Design review of the part built by this model. Coordinates are the model's own, in mm. A direction names the side the tool comes from. Round coordinates to 2 decimals unless told otherwise and drop trailing zeros. Loops run counter-clockwise (first coordinate to the right, second up) from the corner with the lowest first, then second, coordinate; pieces in that order, holes last. Notation, with made-up numbers: (-16.75, 65) - (5.25, 65) arc R32 cw to (5.25, 103) - close; hole circle Ø5 at (-1, 3). An arc over 180 degrees is marked (long way). Answer as CSV lines item,"result". Start each with the question number.
(1) Consider section A-A (z = -13.5). Give the boundary of the cut face in (x, y).
(2) For P1, Ø1.5, axis at x = 1.5, z = 3, coming from the +Y side; P2, Ø3, axis at y = 8.5, z = -5.5, coming from the -X side; P3, Ø1, axis at x = 2, y = -10.5, coming from the +Z side, all flat-tipped, find the tip position at first contact; note any pin that passes through.
(3) For faces 1 (the cylindrical face through (1.726, 1.21, -14.815)), 2 (the cylindrical face through (1.726, -14.464, 3.427)), 3 (the cylindrical face through (2, -14, 6)), 4 (the cylindrical face through (2, 6, 14)), list the 3-axis set-ups (+Z, -Z, +X, -X, +Y, -Y) from which the entire face can be reached by the end or side of a thin tool; tool diameter is ignored.
(4) Consider section C-C (z = 6). Give the boundary of the cut face in (x, y), and give its area (3 significant figures).
(5) Wall thickness on L1, parallel to Y at x = 1.8, z = 14; L2, parallel to Z at x = 3.1, y = -11: over which ranges is each line inside the solid? List them lowest first.
(6) Mouldability with a two-part tool opening along Y and no side actions: class faces 5 (the cylindrical face through (2, -14, -6)), 6 (the cylindrical face through (1.73, 7.74, -12.75)) as released by +Y, released by -Y, zero draft, split by the parting line, or undercut.
(7) Consider section B-B (y = -14). Give the boundary of the cut face in (x, z), and give its area (3 significant figures).
(8) Consider section D-D (y = -9.5). Give the boundary of the cut face in (x, z).
from build123d import *

# Parameters (mm, degrees)
BASPROSKE_W        = 3.5
BASPROSKE_H        = 16.5
TOOTHCUT_DEPTH     = 24.595550428
TEETHCUTS_COUNT    = 20
TEETHCUTS_ANGLE    = 342
BORSKE_R           = 0.5
BORE_DEPTH         = 50.0000508
CUT_EXTRUDE1_DEPTH = 10


with BuildPart() as part:
    # BasProSke → Base-Revolve (revolve)
    with BuildSketch(Plane(origin=(0, 0, 0), x_dir=(1, 0, 0), z_dir=(0, 1, 0)), mode=Mode.PRIVATE) as base_revolve_sk:
        with Locations((1.75, 8.25)):
            Rectangle(BASPROSKE_W, BASPROSKE_H)
    revolve(base_revolve_sk.sketch.rotate(Axis((-10, 0, 0), (1, 0, 0)), 180), axis=Axis((-10, 0, 0), (1, 0, 0)))

    # TooCutSke → ToothCut (cut, through all)
    with BuildSketch(Plane(origin=(0, 0, 0), x_dir=(0, 0, -1), z_dir=(1, 0, 0))):
        with BuildLine():
            ThreePointArc((0.74381438, 13.102904875), (0, 13.124), (-0.74381438, 13.102904875))
            ThreePointArc((-0.74381438, 13.102904875), (-1.226473103, 14.852072512), (-2.209965745, 16.376962373))
            ThreePointArc((-2.209965745, 16.376962373), (0, 16.5254), (2.209965745, 16.376962373))
            ThreePointArc((2.209965745, 16.376962373), (1.226473103, 14.852072512), (0.74381438, 13.102904875))
        make_face()
    toothcut = extrude(amount=TOOTHCUT_DEPTH, mode=Mode.SUBTRACT)

    # TeethCuts: ToothCut ×20 about axis
    teethcuts_axis = Axis((-10, 0, 0), (1, 0, 0))
    for i in range(1, TEETHCUTS_COUNT):
        add(toothcut.rotate(teethcuts_axis, i * TEETHCUTS_ANGLE / (TEETHCUTS_COUNT - 1)), mode=Mode.SUBTRACT)

    # BorSke → Bore (cut, symmetric)
    with BuildSketch(Plane(origin=(0, 0, 0), x_dir=(0, 0, -1), z_dir=(1, 0, 0))):
        with Locations(Location((0, 0, 0), (0, 0, 180))):
            Circle(BORSKE_R)
    extrude(amount=BORE_DEPTH, both=True, mode=Mode.SUBTRACT)

    # Sketch1 → Cut-Extrude1 (cut)
    with BuildSketch(Plane.ZY):
        Polygon((-1.083959973, 0.232340082), (-1.46991278, -0.097897743), (-1.664721638, 0.37121429), (-2.099317612, 0.190738968), (-1.908578644, 0), (-2.267755891, -0.359177248), (-1.815166156, -0.589783236), (-2.045772144, -1.042372971), (-1.544072558, -1.12183438), (-1.623533966, -1.623533966), (-1.12183438, -1.544072558), (-1.042372971, -2.045772144), (-0.589783236, -1.815166156), (-0.359177248, -2.267755891), (0, -1.908578644), (0.359177248, -2.267755891), (0.589783236, -1.815166156), (1.042372971, -2.045772144), (1.12183438, -1.544072558), (1.623533966, -1.623533966), (1.544072558, -1.12183438), (2.045772144, -1.042372971), (1.815166156, -0.589783236), (2.267755891, -0.359177248), (1.908578644, 0), (2.267755891, 0.359177248), (1.815166156, 0.589783236), (2.045772144, 1.042372971), (1.544072558, 1.12183438), (1.623533966, 1.623533966), (1.182876639, 1.553740702), (0.828023136, 1.406380155), (1.022831994, 0.937268122), (0.516480691, 0.896957479), (0.556791334, 0.390606175), (0.062765954, 0.508739633), (-0.055367504, 0.014714252), (-0.488708315, 0.279728085), (-0.753722148, -0.153612726), align=None)
    extrude(amount=-CUT_EXTRUDE1_DEPTH, mode=Mode.SUBTRACT)


solid = part.part
Determined:
1,outline,"(0, -7.85) - (3.5, -7.85) - (3.5, -5.55) - (0, -5.55) - close; (0, -3.45) - (3.5, -3.45) - (3.5, -0.8) - (0, -0.8) - close; (0, 0.8) - (3.5, 0.8) - (3.5, 3.45) - (0, 3.45) - close; (0, 5.55) - (3.5, 5.55) - (3.5, 7.85) - (0, 7.85) - close"
2,P1,"stops at y = 16.35"
2,P2,"stops at x = 0"
2,P3,"stops at z = 11.84"
3,face 1,"-Z, +X, -X"
3,face 2,"+X, -X"
3,face 3,"+X, -X, -Y"
3,face 4,"+Z, +X, -X"
4,outline,"(0, -14) - (3.5, -14) - (3.5, 14) - (0, 14) - close"
4,area,"98.0 mm^2"
5,L1,"y = -7.87 to -6, -3.46 to -0.92, 0.92 to 3.46, 6 to 7.87"
5,L2,"z = -11.84 to -9.26, -7.16 to 7.16, 9.26 to 11.84"
6,face 5,"released by -Y"
6,face 6,"undercut"
7,outline,"(0, -7.87) - (3.5, -7.87) - (3.5, -6) - (0, -6) - close; (0, -3.46) - (3.5, -3.46) - (3.5, -0.92) - (0, -0.92) - close; (0, 0.92) - (3.5, 0.92) - (3.5, 3.46) - (0, 3.46) - close; (0, 6) - (3.5, 6) - (3.5, 7.87) - (0, 7.87) - close"
7,area,"30.8 mm^2"
8,outline,"(0, -11.16) - (3.5, -11.16) - (3.5, 11.16) - (0, 11.16) - close"
